Build history of the part. All positions in model axes, mm. A direction names the side the tool comes from. Round coordinates to 2 decimals unless told otherwise and drop trailing zeros. Loops run counter-clockwise (first coordinate to the right, second up) from the corner with the lowest first, then second, coordinate; pieces in that order, holes last. Notation, with made-up numbers: M -20,-2 L 37,-2 A24 cw 37,14 Z; hole C 8,31 d7. An arc over 180 degrees is marked long. Use one line per item in the form item = value. Start each with the question number.
```python
from build123d import *

# Parameters (mm, degrees)
SKETCH2_R                = 254
BOSS_EXTRUDE2_DEPTH      = 1905
BOSS_EXTRUDE3_DEPTH      = 63.5
BOSS_EXTRUDE3_DEPTH_BACK = 1968.5
SKETCH3_R                = 88.9
FILLET1_R                = 12.7
SKETCH4_R                = 38.1
CUT_EXTRUDE1_DEPTH       = 7.62
CUT_EXTRUDE2_START       = -7.62
SKETCH5_R                = 38.1
CUT_EXTRUDE2_DEPTH       = 7.62


with BuildPart() as part:
    # Sketch2 → Boss-Extrude2 (new body)
    with BuildSketch(Plane.XY):
        Circle(SKETCH2_R)
    extrude(amount=BOSS_EXTRUDE2_DEPTH)

    # Sketch3 → Boss-Extrude3 (add, two sides: drawn at the far end of the back side and taken through both)
    with BuildSketch(Plane.XY.offset(1905).offset(-BOSS_EXTRUDE3_DEPTH_BACK)):
        Circle(SKETCH3_R)
    extrude(amount=BOSS_EXTRUDE3_DEPTH + BOSS_EXTRUDE3_DEPTH_BACK)

    # Fillet1
    fillet1_edges = [part.edges().sort_by_distance(p)[0] for p in [
        (-88.9, 0, -63.5),
        (-88.9, 0, 1968.5),
    ]]
    fillet(fillet1_edges, radius=FILLET1_R)

    # Sketch4 → Cut-Extrude1 (cut)
    with BuildSketch(Plane(origin=(0, 0, -63.5), x_dir=(-1, 0, 0), z_dir=(0, 0, -1))):
        Circle(SKETCH4_R)
    extrude(amount=-CUT_EXTRUDE1_DEPTH, mode=Mode.SUBTRACT)

    # Sketch5 → Cut-Extrude2 (cut)
    with BuildSketch(Plane.XY.offset(1968.5).offset(CUT_EXTRUDE2_START)):
        with Locations(Location((0, 0, 0), (0, 0, 180))):
            Circle(SKETCH5_R)
    extrude(amount=CUT_EXTRUDE2_DEPTH, mode=Mode.SUBTRACT)


solid = part.part
```
Q1. Saw through at D-D (y = -155). Give the cut face in (x, z).
Q2. Tool access for faces 4 (the face through (84.795, 26.703, -25.756)), 5 (the face through (16, 35, 1968.5)), 6 (the face through (1, -1, 1960.88)): list every direction of +Z, -Z, +X, -X, +Y, -Y with a clear straight run to the whole face (end or side of a thin tool).
Q3. Saw through at A-A (y = 0). Give the cut face in (x, z).
Q4. Drop flat-ended pins along their axis: P1, Ø4, axis at x = 145, y = -169.5, coming from the +Z side; P2, Ø6, axis at y = 173, z = 767.5, coming from the +X side; P3, Ø1, axis at x = -170, z = 227, coming from the -Y side. Give the stop position or say it passes through.
Q5. Wall check: probe 1 along Z at (x, y) = (-116.5, 163.5); probe 2 along Y at (x, z) = (0, 1966.25); probe 3 along Y at (x, z) = (0, -59). Give the ranges that are in metal, low to high.
Q6. Saw through at C-C (z = 251.5). Give the cut face in (x, y).
Q7. Pull direction X, two halves, no side cores. Call faces 1 (the face through (-55.06, -247.96, 939.16)), 2 (the face through (16, 35, -63.5)), 3 (the face through (30.235, -23.183, -59.743)): pulls with the +X half, pulls with the -X half, needs draft (parallel to the pull), parting line crosses it, or undercut.
Filled in:
q1.outline = M -201.22,0 L 201.22,0 L 201.22,1905 L -201.22,1905 Z
q2.face_4 = -Z
q2.face_5 = +Z, +X, -X, +Y, -Y
q2.face_6 = +Z
q3.outline = M -254,0 L -88.9,0 L -88.9,-50.8 A12.7 ccw -76.2,-63.5 L -38.1,-63.5 L -38.1,-55.88 L 38.1,-55.88 L 38.1,-63.5 L 76.2,-63.5 A12.7 ccw 88.9,-50.8 L 88.9,0 L 254,0 L 254,1905 L 88.9,1905 L 88.9,1955.8 A12.7 ccw 76.2,1968.5 L 38.1,1968.5 L 38.1,1960.88 L -38.1,1960.88 L -38.1,1968.5 L -76.2,1968.5 A12.7 ccw -88.9,1955.8 L -88.9,1905 L -254,1905 Z
q4.P1 = 1905
q4.P2 = 188.72
q4.P3 = -189.17
q5.probe_1 = 0 to 1905
q5.probe_2 = -83.42 to -38.1, 38.1 to 83.42
q5.probe_3 = -85.9 to -38.1, 38.1 to 85.9
q6.outline = C 0,0 d508
q7.face_1 = parting line crosses it
q7.face_2 = needs draft
q7.face_3 = undercut
